Autodesk Inventor part; units mm, degrees
ref_plane "YZ Plane" through (0, 0, 0) normal (1, 0, 0) x (0, 1, 0)
ref_plane "XZ Plane" through (0, 0, 0) normal (0, 1, 0) x (-1, 0, 0)
ref_plane "XY Plane" through (0, 0, 0) normal (0, 0, 1) x (1, 0, 0)
sketch "Náčrt1" plane through (0, 0, 0) normal (0, 1, 0) x (-1, 0, 0)
  line L0 (0, 0) -> (50, 0)
  line L1 (50, 0) -> (66.0697, -19.1511)
  line L2 (50, 0) -> (75, 0) construction
  line L3 (66.0697, -19.1511) -> (58.4092, -25.579)
  line L4 (0, -12) -> (0, 0)
  line L5 (58.6554, -25.3724) -> (47.4347, -12)
  line L6 (47.4347, -12) -> (0, -12)
  dimension "d0" = 50
  dimension "d2" = 25
  dimension "d3" = 50
  dimension "d4" = 10
  dimension "d5" = 12
extrude "Vysunutí1" add sketch "Náčrt1" along normal blind 15
sketch "Náčrt8" plane through (-66.0697, 0, -19.1511) normal (-0.6428, 0, -0.766) x (-0.766, 0, 0.6428)
  line L0 (-9.6786, 0) -> (-9.6786, 15)
  line L1 (-9.6786, 7.5) -> (0, 7.5)
  line L2 (0, 0) -> (0, 15)
  point P0 (-38.3022, 0)
sketch "Náčrt9" plane through (-50, 0, 0) normal (-0.766, 0, 0.6428) x (0.6428, 0, 0.766)
  line L0 (-25, 0) -> (-25, 15)
  line L1 (0, 0) -> (0, 15)
sketch "Náčrt10" plane through (-50, 0, 0) normal (0, 0, 1) x (1, 0, 0)
  line L0 (0, 0) -> (0, 15)
  line L1 (0, 7.5) -> (50, 7.5)
  line L2 (50, 0) -> (50, 15)
sketch "Náčrt11" plane through (0, 0, 0) normal (1, 0, 0) x (0, 0, -1)
  line L0 (0, 0) -> (0, 15)
  line L1 (0, 7.5) -> (12, 7.5)
  line L2 (12, 0) -> (12, 15)
  line L3 (0, 3.5) -> (4, 3.5)
  line L4 (4, 3.5) -> (4, 11.5)
  line L5 (4, 11.5) -> (0, 11.5)
  line L6 (0, 11.5) -> (0, 3.5)
  point P0 (0, 7.5)
  point P1 (0, 11.5)
  dimension "d64" = 4
  dimension "d65" = 8
extrude "Vysunutí10" cut sketch "Náčrt11" against normal through all
sketch "Náčrt21" plane through (-66.0697, 0, -19.1511) normal (-0.6428, 0, -0.766) x (-0.766, 0, 0.6428)
  line L0 (0, 0) -> (0, 15)
  line L1 (0, 3.5) -> (-4, 3.5)
  line L2 (-4, 3.5) -> (-4, 11.5)
  line L3 (-4, 11.5) -> (0, 11.5)
  line L4 (0, 11.5) -> (0, 3.5)
  point P0 (-38.3022, 0)
  point P1 (0, 7.5)
  point P2 (0, 11.5)
  dimension "d68" = 4
  dimension "d69" = 8
extrude "Vysunutí11" cut sketch "Náčrt21" against normal through all
sketch "Náčrt22" plane through (-63.0055, 3.5, -21.7223) normal (-0.766, 0, 0.6428) x (0.6428, 0, 0.766)
  line L0 (0, -3.5) -> (0, 11.5)
  line L1 (0, 4) -> (23.1348, 4)
  line L2 (23.1348, 8) -> (23.1348, 0)
  circle A0 centre (7.71, 4) radius 2.8
  point P0 (57.1394, -3.5)
  dimension "d72" = 5.6
sketch "Náčrt25" plane through (-58.6554, 0, -25.3724) normal (-0.6428, 0, -0.766) x (-0.766, 0, 0.6428)
  line L0 (5.6786, 3.5) -> (5.6786, 11.5)
  line L1 (5.6786, 5.4735) -> (0, 5.4735)
  line L2 (0, 0) -> (0, 15)
  point P0 (-28.6236, 0)
  dimension "d73" = 5.6786
extrude "Vysunutí12" cut sketch "Náčrt22" against normal blind 2
sketch "Náčrt27" plane through (-56.5175, 7.5, -17.1016) normal (-0.766, 0, 0.6428) x (0.6428, 0, 0.766)
  circle A0 centre (0, 0) radius 2.8
  line L0 (0, -2.8) -> (0, 2.8)
  line L1 (-2.7895, 0) -> (2.8105, 0)
  circle A1 centre (0, 0) radius 2.45
  point P0 (49.4294, -7.5)
  dimension "d79" = 5.6
  dimension "d80" = 4.9
extrude "Vysunutí14" cut sketch "Náčrt27" against normal through all contours A1 L0 L1 | L1 L0 A1 | L0 L1 A1 | A1 L1 L0
sketch "Náčrt28" plane through (0, 0, 0) normal (1, 0, 0) x (0, 0, -1)
  line L0 (0, 0) -> (0, 3.5)
  line L1 (12, 0) -> (12, 15)
  line L2 (0, 0) -> (12, 0)
  line L3 (0, 15) -> (12, 15)
  line L4 (0, 11.5) -> (0, 15)
  line L5 (1, 0.6751) -> (10, 0.6751)
  line L6 (4, 11.5) -> (4, 3.5)
  line L7 (1, 2.8249) -> (5, 2.8249)
  line L8 (1, 12.1751) -> (5, 12.1751)
  line L9 (1, 14.3249) -> (10, 14.3249)
  line L10 (5, 2.8249) -> (5, 12.1751)
  line L11 (9.8978, 0.6751) -> (9.8978, 14.3249)
  line L12 (1, 0.6751) -> (1, 2.8249)
  line L13 (1, 12.1751) -> (1, 14.3249)
  line L14 (4, 7.5) -> (12, 7.5)
  point P0 (5, 7.5)
  point P1 (9.8978, 7.5)
  point P2 (5.5, 0.6751)
  point P3 (5.5, 14.3249)
  point P4 (1, 13.25)
  point P5 (0, 13.25)
  point P6 (1, 1.75)
  point P7 (0, 1.75)
extrude "Vysunutí15" add sketch "Náčrt28" along normal blind 10
properties part number "LAMPA1"
Work out the finished part from the listing and answer in its coordinate system (mm). A direction names the side the tool comes from. Coordinates: 2 decimals unless noted, no trailing zeros. Write each loop counter-clockwise with the first axis right and the second up, starting at its lowest first coordinate (ties: lowest second). Pieces come first, ordered by that corner, then holes.
Q1. A cutting plane is placed at C-C, the plane y = 13.5. Give the vertices of the cut face in (x, z).
Q2. Which of the six approach directions +Z, -Z, +X, -X, +Y, -Y give full straight-line access (tool end or side, diameter ignored) to faces 5 (the face through (5, 7, -9.898)), 6 (the face through (5, 14.325, -5)), 7 (the face through (5, 2.825, -3)), 8 (the face through (-55.674, 7.444, -12.985))?
Q3. A cutting plane is placed at A-A, the plane x = -11. Give the vertices of the cut face in (y, z).
Q4. Find the intervals of material crossed by line 1 (Y direction, x = -31.5, z = -3.5); line 2 (Z direction, x = -6.5, y = 10); line 3 (Z direction, x = -33.5, y = 13.25), in increasing order.
Q5. Each of these flat-tipped pins is pushed along its axis until it touches: pin 1 Ø9 at (x, y) = (-18.5, 8.5) entering from +Z; pin 2 Ø2.5 at (x, z) = (7, -3.5) entering from -Y; pin 3 Ø4 at (x, y) = (-26.5, 7.5) entering from +Z; pin 4 Ø1.1 at (x, y) = (4, 1.5) entering from +Z. Where does it stop, or does it pass through?
Q6. A cutting plane is placed at D-D, the plane z = -6. Give the vertices of the cut face in (x, y).
Q7. Determine the mould class of faces 1 (the face through (-25, 2, 0)), 2 (the face through (-33, 15, -7)), 3 (the face through (-51.877, 7.395, -17.294)), 4 (the face through (-58.722, 5.796, -18.153)) for opening direction Z: released by +Z, released by -Z, zero draft, split by the parting line, or undercut.
Q8. A cutting plane is placed at B-B, the plane z = -2. Give the vertices of the cut face in (x, y), then the cut area to 3 significant figures.
Findings below:
1. outline: (-66.07, -19.15) - (-58.66, -25.37) - (-47.43, -12) - (0, -12) - (0, -9.9) - (10, -9.9) - (10, -1) - (0, -1) - (0, 0) - (-50, 0) - close
2. face 5: -Z, +X, +Y, -Y
2. face 6: +Z, -Z, +X, +Y
2. face 7: +Z, +X
2. face 8: +Z, -X
3. outline: (0, -12) - (15, -12) - (15, 0) - (11.5, 0) - (11.5, -4) - (3.5, -4) - (3.5, 0) - (0, 0) - close
4. line 1: y = 0 to 3.5, 11.5 to 15
4. line 2: z = -12 to -4
4. line 3: z = -12 to 0
5. pin 1: stops at z = 0
5. pin 2: stops at y = 0.68
5. pin 3: stops at z = -4
5. pin 4: stops at z = -1
6. outline: (-55.03, 0) - (0, 0) - (0, 0.68) - (10, 0.68) - (10, 14.32) - (0, 14.32) - (0, 15) - (-55.03, 15) - (-55.03, 11.5) - (-49.81, 11.5) - (-49.81, 3.5) - (-55.03, 3.5) - close
7. face 1: released by +Z
7. face 2: zero draft
7. face 3: released by -Z
7. face 4: undercut
8. outline: (-51.68, 0) - (0, 0) - (0, 0.68) - (10, 0.68) - (10, 2.82) - (0, 2.82) - (0, 3.5) - (-51.68, 3.5) - close; (-51.68, 11.5) - (0, 11.5) - (0, 12.18) - (10, 12.18) - (10, 14.32) - (0, 14.32) - (0, 15) - (-51.68, 15) - close
8. area: 405 mm2
